```python
from build123d import *

# Parameters (mm, degrees)
BOSS_EXTRUDE1_DEPTH     = 6.35
BOSS_EXTRUDE3_DEPTH     = 25.4
CUT_EXTRUDE1_DEPTH      = 263.978228947
CUT_EXTRUDE1_DEPTH_BACK = 263.978228947
SKETCH2_R               = 39.05


with BuildPart() as part:
    # Sketch1 → Boss-Extrude1 (new, symmetric)
    with BuildSketch(Plane(origin=(0, 0, 0), x_dir=(1, 0, 0), z_dir=(0, 1, 0))):
        with BuildLine():
            Line((95.25, -51.587287188), (95.25, -42.12))
            Line((95.25, -42.12), (95.25, 42.12))
            Line((95.25, 42.12), (95.25, 51.587287188))
            ThreePointArc((95.25, 51.587287188), (93.136460997, 55.353844077), (90.531290228, 58.798707381))
            ThreePointArc((90.531290228, 58.798707381), (51.506708486, 94.86970792), (0, 107.95))
            ThreePointArc((0, 107.95), (-52.123153766, 100.419362872), (-99.983255054, 78.443367814))
            ThreePointArc((-99.983255054, 78.443367814), (-137.771381999, 62.338580791), (-178.772455636, 59.844855919))
            ThreePointArc((-178.772455636, 59.844855919), (-198.978805326, 51.581494612), (-208.83628251, 32.103048795))
            ThreePointArc((-208.83628251, 32.103048795), (-124.636067917, -68.271246819), (0.22501695, -107.949765481))
            ThreePointArc((0.22501695, -107.949765481), (51.605556398, -94.81597465), (90.531290228, -58.798707381))
            ThreePointArc((90.531290228, -58.798707381), (93.136460997, -55.353844077), (95.25, -51.587287188))
        make_face()
    extrude(amount=BOSS_EXTRUDE1_DEPTH, both=True)

    # Sketch1_4 → Boss-Extrude3 (add, symmetric)
    with BuildSketch(Plane(origin=(0, 0, 0), x_dir=(1, 0, 0), z_dir=(0, 1, 0))):
        with BuildLine():
            Line((114.3, -55.358016583), (114.3, 55.358016583))
            ThreePointArc((114.3, 55.358016583), (110.69531577, 63.1385236), (105.833333333, 70.201891396))
            ThreePointArc((105.833333333, 70.201891396), (60.055640005, 111.903172894), (0, 127))
            ThreePointArc((0, 127), (-57.515204156, 118.690331445), (-110.326350404, 94.440957588))
            ThreePointArc((-110.326350404, 94.440957588), (-142.699370878, 80.750483212), (-177.8, 78.91))
            ThreePointArc((-177.8, 78.91), (-213.353328958, 64.183328958), (-228.08, 28.63))
            ThreePointArc((-228.08, 28.63), (-137.03440171, -82.883921429), (0, -127))
            ThreePointArc((0, -127), (60.055640005, -111.903172894), (105.833333333, -70.201891396))
            ThreePointArc((105.833333333, -70.201891396), (110.69531577, -63.1385236), (114.3, -55.358016583))
        make_face()
        with BuildLine():
            Line((95.25, 42.12), (95.25, -42.12))
            Line((95.25, -42.12), (95.25, -51.587287188))
            ThreePointArc((95.25, -51.587287188), (93.136460997, -55.353844077), (90.531290228, -58.798707381))
            ThreePointArc((90.531290228, -58.798707381), (51.605556398, -94.81597465), (0.22501695, -107.949765481))
            ThreePointArc((0.22501695, -107.949765481), (-124.636067917, -68.271246819), (-208.83628251, 32.103048795))
            ThreePointArc((-208.83628251, 32.103048795), (-198.978805326, 51.581494612), (-178.772455636, 59.844855919))
            ThreePointArc((-178.772455636, 59.844855919), (-137.771381999, 62.338580791), (-99.983255054, 78.443367814))
            ThreePointArc((-99.983255054, 78.443367814), (-52.123153766, 100.419362872), (0, 107.95))
            ThreePointArc((0, 107.95), (51.506708486, 94.86970792), (90.531290228, 58.798707381))
            ThreePointArc((90.531290228, 58.798707381), (93.136460997, 55.353844077), (95.25, 51.587287188))
            Line((95.25, 51.587287188), (95.25, 42.12))
        make_face(mode=Mode.SUBTRACT)
    extrude(amount=BOSS_EXTRUDE3_DEPTH, both=True)

    # Sketch2 → Cut-Extrude1 (cut, two sides: drawn at the far end of the back side and taken through both)
    with BuildSketch(Plane(origin=(0, 6.35, 0), x_dir=(1, 0, 0), z_dir=(0, 1, 0)).offset(-CUT_EXTRUDE1_DEPTH_BACK)):
        with Locations(Location((0, 0, 0), (0, 0, 270))):
            Circle(SKETCH2_R)
    extrude(amount=CUT_EXTRUDE1_DEPTH + CUT_EXTRUDE1_DEPTH_BACK, mode=Mode.SUBTRACT)


solid = part.part
```
Could you check a few things on this model? Use its own coordinates, in mm. A direction names the side the tool comes from. Round coordinates to 2 decimals unless told otherwise and drop trailing zeros. Write each loop counter-clockwise with the first axis right and the second up, starting at its lowest first coordinate (ties: lowest second). Pieces come first, ordered by that corner, then holes. Notation, with made-up numbers: M -26,-14 L -10,-14 A20 cw -10,-7 Z; hole C 47,66.25 d9. An arc over 180 degrees is marked long. Write each question's results on one line, items separated by ' | '. Start each with the question number.
1. I'm going to push flat-ended pins straight in: pin 1 Ø2 at (y, z) = (-2, -87.5) entering from +X; pin 2 Ø10 at (y, z) = (-19.5, 58) entering from -X; pin 3 Ø3 at (x, z) = (-2.5, -98) entering from -Y. Where does each tip first touch, or does it pass through?
2. Thinking about a two-plate mould opening in X: for faces 1 (the face through (60.8, 0.4, -111.5)), 2 (the face through (-70, -25.4, -95)), 3 (the face through (93.103, 16.008, -55.404)), 4 (the face through (-138.718, 0.356, 81.725)), which applies, +X half, -X half, draft (parallel to the pull), parting line (faces both ways), or undercut?
3. Imagine slicing it at B-B on z = 0. List the corners of the cut face in (x, y) for me, and give its area (3 significant figures).
4. I need wall thicknesses on L1, parallel to Z at x = 67, y = 1.5; L2, parallel to X at y = -9.5, z = 19; L3, parallel to Y at x = -71.5, z = 16.5. Which ranges of each line are inside material? Lowest first, please. Write a range as from..to.
5. On a 3-axis mill with a long thin cutter (end or side, diameter ignored), from which of +Z, -Z, +X, -X, +Y, -Y can I reach the whole of each face in a straight line? I mean faces 5 (the face through (-138.33, 16.01, -62.21)), 6 (the face through (-52.83, -15.74, -100.21)), 7 (the face through (-142.22, 0.36, -80.86)). Say none if no direction works.
6. Imagine slicing it at D-D on x = -78.5. List the corners of the cut face in (y, z) for me, and give its area (3 significant figures).
7. Imagine slicing it at C-C on x = -182.5. List the corners of the cut face in (y, z) for me, and give its area (3 significant figures).
8. Imagine slicing it at A-A on y = 13. List the corners of the cut face in (x, z) for me.
Result sheet:
1) pin 1: stops at x = 92.99 | pin 2: stops at x = -173.15 | pin 3: stops at y = -6.35
2) face 1: +X half | face 2: draft | face 3: undercut | face 4: -X half
3) outline: M -213.88,-25.4 L -191.59,-25.4 L -191.59,-6.35 L -39.05,-6.35 L -39.05,6.35 L -191.59,6.35 L -191.59,25.4 L -213.88,25.4 Z; M 39.05,-6.35 L 95.25,-6.35 L 95.25,-25.4 L 114.3,-25.4 L 114.3,25.4 L 95.25,25.4 L 95.25,6.35 L 39.05,6.35 Z | area: 4,750 mm^2
4) L1: z = -107.89..107.89 | L2: x = -201.77..-178.01, 95.25..114.3 | L3: y = -6.35..6.35
5) face 5: +Y | face 6: -Y | face 7: -Z, +Y, -Y
6) outline: M -25.4,-111.22 L 25.4,-111.22 L 25.4,-90.38 L 6.35,-90.38 L 6.35,92.25 L 25.4,92.25 L 25.4,112.56 L -25.4,112.56 L -25.4,92.25 L -6.35,92.25 L -6.35,-90.38 L -25.4,-90.38 Z | area: 4,410 mm^2
7) outline: M -25.4,-78.69 L 25.4,-78.69 L 25.4,-59.5 L 6.35,-59.5 L 6.35,13.15 L 25.4,13.15 L 25.4,43.18 L -25.4,43.18 L -25.4,13.15 L -6.35,13.15 L -6.35,-59.5 L -25.4,-59.5 Z | area: 3,420 mm^2
8) outline: M -228.08,-28.63 A50.28 ccw -177.8,-78.91 A101.6 cw -110.33,-94.44 A203.2 ccw 0,-127 A127 ccw 105.83,-70.2 A50.8 ccw 114.3,-55.36 L 114.3,55.36 A50.8 ccw 105.83,70.2 A127 ccw 0,127 A254 ccw Z; hole M -208.84,-32.1 A31.23 ccw -178.77,-59.84 A120.65 cw -99.98,-78.44 A184.15 ccw 0,-107.95 A107.95 ccw 90.53,-58.8 A31.75 ccw 95.25,-51.59 L 95.25,51.59 A31.75 ccw 90.53,58.8 A107.95 ccw 0.23,107.95 A234.95 ccw Z
